Could you check a few things on this model? Use its own coordinates, in mm. Give positions to 0.01 mm unless a question says otherwise; leave off trailing zeros. Write each loop counter-clockwise with the first axis right and the second up, starting at its lowest first coordinate (ties: lowest second). Pieces come first, ordered by that corner, then holes. Notation, with made-up numbers: M -33.75,-11.75 L -17.75,-11.75 A18 cw -17.75,-1.75 Z; hole C -23.75,-35 d4. An arc over 180 degrees is marked long. One line per item, written item: value.
```python
from build123d import *

# Parameters (mm, degrees)
SKETCH1_W               = 466
SKETCH1_H               = 126.5
BOSS_EXTRUDE1_DEPTH     = 6
SKETCH2_W               = 73.428571429
SKETCH2_H               = 6
SKETCH2_W_2             = 73.428571428
BOSS_EXTRUDE2_DEPTH     = 20
SKETCH1_2_W             = 466
SKETCH1_2_H             = 126.5
CUT_EXTRUDE1_DEPTH      = 7
CUT_EXTRUDE1_DEPTH_BACK = 15
SKETCH2_4_W             = 73.428571429
SKETCH2_4_H             = 6
BOSS_EXTRUDE3_DEPTH     = 6
SKETCH4_W               = 6
SKETCH4_H               = 6.666666666
BOSS_EXTRUDE4_DEPTH     = 6


with BuildPart() as part:
    # Sketch1 → Boss-Extrude1 (new body)
    with BuildSketch(Plane(origin=(0, 0, 0), x_dir=(1, 0, 0), z_dir=(0, 1, 0))):
        Rectangle(SKETCH1_W, SKETCH1_H)
    extrude(amount=BOSS_EXTRUDE1_DEPTH)

    # Sketch1<2> → Cut-Extrude1 (cut, two sides)
    with BuildSketch(Plane(origin=(0, 0, 0), x_dir=(1, 0, 0), z_dir=(0, 1, 0))) as cut_extrude1_sk:
        Rectangle(SKETCH1_2_W, SKETCH1_2_H)
    extrude(amount=CUT_EXTRUDE1_DEPTH, mode=Mode.SUBTRACT)
    extrude(cut_extrude1_sk.sketch, amount=-CUT_EXTRUDE1_DEPTH_BACK, mode=Mode.SUBTRACT)


with BuildPart() as body_2:
    # Sketch2 → Boss-Extrude2 (new body)
    with BuildSketch(Plane(origin=(0, 6, 0), x_dir=(1, 0, 0), z_dir=(0, 1, 0))):
        with Locations((-220.285714286, 90.25)):
            Rectangle(SKETCH2_W, SKETCH2_H)
        with Locations((-146.857142857, 90.25)):
            Rectangle(SKETCH2_W_2, SKETCH2_H)
        with Locations((-73.428571428, 90.25)):
            Rectangle(SKETCH2_W, SKETCH2_H)
        with Locations((0, 90.25)):
            Rectangle(SKETCH2_W_2, SKETCH2_H)
        with Locations((73.428571428, 90.25)):
            Rectangle(SKETCH2_W, SKETCH2_H)
        with Locations((146.857142857, 90.25)):
            Rectangle(SKETCH2_W_2, SKETCH2_H)
        with Locations((220.285714286, 90.25)):
            Rectangle(SKETCH2_W, SKETCH2_H)
    extrude(amount=-BOSS_EXTRUDE2_DEPTH)

    # Sketch2<4> → Boss-Extrude3 (add)
    with BuildSketch(Plane(origin=(0, 6, 0), x_dir=(1, 0, 0), z_dir=(0, 1, 0))):
        with Locations((220.285714286, 90.25)):
            Rectangle(SKETCH2_4_W, SKETCH2_4_H)
        with Locations((73.428571428, 90.25)):
            Rectangle(SKETCH2_4_W, SKETCH2_4_H)
        with Locations((-73.428571428, 90.25)):
            Rectangle(SKETCH2_4_W, SKETCH2_4_H)
        with Locations((-220.285714286, 90.25)):
            Rectangle(SKETCH2_4_W, SKETCH2_4_H)
    extrude(amount=BOSS_EXTRUDE3_DEPTH)

    # Sketch4 → Boss-Extrude4 (add)
    with BuildSketch(Plane.ZY.offset(257)):
        with Locations((-90.25, -4)):
            Rectangle(SKETCH4_W, SKETCH4_H)
    boss_extrude4 = extrude(amount=BOSS_EXTRUDE4_DEPTH)

    # Mirror2: Boss-Extrude4 across plane
    add(boss_extrude4.mirror(Plane(origin=(0, 0, 0), x_dir=(0, 0, 1), z_dir=(1, 0, 0))))


solid = body_2.part
```
1) If we section it at B-B, the plane x = -12: Write out the boundary of the cut face in (y, z).
Outcome:
outline: M -14,-93.25 L 6,-93.25 L 6,-87.25 L -14,-87.25 Z
2) If we section it at A-A, the plane z = -90.25: Write out the boundary of the cut face in (x, y).
Outcome:
outline: M -263,-7.33 L -257,-7.33 L -257,-14 L 257,-14 L 257,-7.33 L 263,-7.33 L 263,-0.67 L 257,-0.67 L 257,12 L 183.57,12 L 183.57,6 L 110.14,6 L 110.14,12 L 36.71,12 L 36.71,6 L -36.71,6 L -36.71,12 L -110.14,12 L -110.14,6 L -183.57,6 L -183.57,12 L -257,12 L -257,-0.67 L -263,-0.67 Z
3) Please list where these lines run through material, in increasing order: L1, parallel to X at y = 6.25, z = -89.1; L2, parallel to Y at x = 30, z = -87.5; L3, parallel to X at y = 2.75, z = -88.1. Write a range as from..to.
Outcome:
L1: x = -257..-183.57, -110.14..-36.71, 36.71..110.14, 183.57..257
L2: y = -14..6
L3: x = -257..257
4) I'm going to push flat-ended pins straight in: pin 1 (1.8 mm diameter, centred on y = 7.5, z = -89, fed in from -X); pin 2 (3 mm diameter, centred on y = -11, z = -92, fed in from +X); pin 3 (3 mm diameter, centred on x = 15, z = -89, fed in from +Y). Where does each tip first touch, or does it pass through?
Outcome:
pin 1: stops at x = -257
pin 2: stops at x = 257
pin 3: stops at y = 6
